```python
from build123d import *

# Parameters (mm, degrees)
F0_R     = 127
F0_R_2   = 12.7
F1_DEPTH = 25.4
F2_W     = 50.8
F2_H     = 50.8
F3_DEPTH = 25.4


with BuildPart() as f1:
    # F0 (on Front) → F1 (new body, symmetric)
    with BuildSketch(Plane.XZ):
        Circle(F0_R)
        Circle(F0_R_2, mode=Mode.SUBTRACT)
    extrude(amount=F1_DEPTH, both=True)

    # F2 (on Front) → F3 (cut, symmetric)
    with BuildSketch(Plane.XZ):
        with Locations((0, 43.010666)):
            Rectangle(F2_W, F2_H)
    extrude(amount=F3_DEPTH, both=True, mode=Mode.SUBTRACT)


solid = f1.part
```
The listing builds one solid part. Answer for the finished solid, in the listing's coordinates (mm). A direction names the side the tool comes from. Coordinates: 2 decimals unless noted, no trailing zeros. Write each loop counter-clockwise with the first axis right and the second up, starting at its lowest first coordinate (ties: lowest second). Pieces come first, ordered by that corner, then holes.
Q1. Section B-B, the plane x = 0 is taken. Write down the section's boundary in (y, z), then the cut area to 3 significant figures.
Returned:
outline: (-25.4, -127) - (25.4, -127) - (25.4, -12.7) - (-25.4, -12.7) - close; (-25.4, 12.7) - (25.4, 12.7) - (25.4, 17.61) - (-25.4, 17.61) - close; (-25.4, 68.41) - (25.4, 68.41) - (25.4, 127) - (-25.4, 127) - close
area: 9,030 mm2
Q2. Section C-C, the plane y = -1.5 is taken. Write down the section's boundary in (x, z).
Returned:
outline: circle Ø254 at (0, 0); hole (-25.4, 17.61) - (25.4, 17.61) - (25.4, 68.41) - (-25.4, 68.41) - close; hole circle Ø25.4 at (0, 0)
Q3. Find the intervals of material crossed by line 1 along Z through (x, y) = (0, -4); line 2 along Z through (x, y) = (-1.5, -15.5); line 3 along X through (y, z) = (15, 53), in increasing order.
Returned:
line 1: z = -127 to -12.7, 12.7 to 17.61, 68.41 to 127
line 2: z = -126.99 to -12.61, 12.61 to 17.61, 68.41 to 126.99
line 3: x = -115.41 to -25.4, 25.4 to 115.41
Q4. Given P1, Ø2, axis at y = 9, z = -51, coming from the +X side; P2, Ø12, axis at y = -19.5, z = 28, coming from the +X side; P3, Ø8, axis at y = 13, z = 50, coming from the -X side, each flat-ended and moving along its own axis, determine where each tip first touches the part or whether it passes through.
Returned:
P1: stops at x = 116.74
P2: stops at x = 125.08
P3: stops at x = -118.38
Q5. Section D-D, the plane z = 40.5 is taken. Write down the section's boundary in (x, y).
Returned:
outline: (-120.37, -25.4) - (-25.4, -25.4) - (-25.4, 25.4) - (-120.37, 25.4) - close; (25.4, -25.4) - (120.37, -25.4) - (120.37, 25.4) - (25.4, 25.4) - close
Q6. Section A-A, the plane z = 0 is taken. Write down the section's boundary in (x, y), then the cut area to 3 significant figures.
Returned:
outline: (-127, -25.4) - (-12.7, -25.4) - (-12.7, 25.4) - (-127, 25.4) - close; (12.7, -25.4) - (127, -25.4) - (127, 25.4) - (12.7, 25.4) - close
area: 11,600 mm2
Q7. Which of the six approach directions +Z, -Z, +X, -X, +Y, -Y give full straight-line access (tool end or side, diameter ignored) to faces 1 (the flat face through (-2, 25.4, -26)), 2 (the flat face through (-25.4, 0, 43))?
Returned:
face 1: +Z, -Z, +X, -X, +Y
face 2: +Y, -Y
Q8. The mould has two halves that part along Z. Classify faces 3 (the flat face through (0, 0, 17.611)), 4 (the flat face through (-2, -25.4, -26)), 5 (the cylindrical face through (-27.53, -0.36, -123.98)): released by +Z, released by -Z, zero draft, split by the parting line, or undercut.
Returned:
face 3: undercut
face 4: zero draft
face 5: split by the parting line
